from build123d import *

# Parameters (mm, degrees)
EXTRUDE_1_DEPTH = 1
SKETCH_2_R      = 3
EXTRUDE_2_DEPTH = 2
SKETCH_3_R      = 3
EXTRUDE_3_DEPTH = 2


with BuildPart() as part:
    # 草图1 → 凸台-拉伸1 (new body)
    with BuildSketch(Plane.XY):
        with BuildLine():
            Line((0, -3.874788925), (-258.053276248, -3.874788925))
            ThreePointArc((-258.053276248, -3.874788925), (-261.928065173, 0), (-258.053276248, 3.874788925))
            Line((-258.053276248, 3.874788925), (0, 3.874788925))
            ThreePointArc((0, 3.874788925), (3.874788925, 0), (0, -3.874788925))
        make_face()
    extrude(amount=EXTRUDE_1_DEPTH)

    # 草图2 → 凸台-拉伸2 (add)
    with BuildSketch(Plane.XY.offset(1)):
        Circle(SKETCH_2_R)
    extrude(amount=EXTRUDE_2_DEPTH)

    # 草图3 → 凸台-拉伸3 (add)
    with BuildSketch(Plane.XY.offset(1)):
        with Locations((-258.053276248, 0)):
            Circle(SKETCH_3_R)
    extrude(amount=EXTRUDE_3_DEPTH)


solid = part.part
Geometry: final body of the model. Coordinates: model frame, mm. A direction names the side the tool comes from. Give positions to 0.01 mm unless a question says otherwise; leave off trailing zeros. Order: outer loops, then holes, each group sorted by start corner. A loop starts at its lowest first (then second) coordinate and runs counter-clockwise, first axis right, second up. Notation, with made-up numbers: (72, 20) -> (95, 20) arc R17 ccw to (95, 24) -> close; hole circle Ø4 at (-37, 71.5). An arc over 180 degrees is marked (long way). Answer as a JSON object with one key per item and string values.
Q1. Material intervals for probe 1 along X at (y, z) = (-0.25, 2.6); probe 2 along Z at (x, y) = (-14, -0.75); probe 3 along X at (y, z) = (-0.25, 0.7), sorted ascending.
Entries:
{"probe 1": "x = -261.04 to -255.06, -2.99 to 2.99", "probe 2": "z = 0 to 1", "probe 3": "x = -261.92 to 3.87"}
Q2. Section C-C (x = -232.5). Output: boundary loops of the cut face in (y, z).
Entries:
{"outline": "(-3.87, 0) -> (3.87, 0) -> (3.87, 1) -> (-3.87, 1) -> close"}
Q3. Draft query along X for faces 3 (the flat face through (-127, 0, 0)), 4 (the cylindrical face through (-3, 0, 2)). Return one class per face: released by +X, released by -X, zero draft, split by the parting line, or undercut.
Entries:
{"face 3": "zero draft", "face 4": "undercut"}
Q4. Access query for faces 1 (the flat face through (0, 0, 3)), 2 (the cylindrical face through (-261.05, 0.13, 1.99)). Directions: +Z, -Z, +X, -X, +Y, -Y. A direction counts if a zero-diameter tool reaches every point of the face in a straight line with its end or side. Return the directions, or none.
Entries:
{"face 1": "+Z, +X, -X, +Y, -Y", "face 2": "+Z"}
Q5. Section B-B (z = 1.55). Output: boundary loops of the cut face in (x, y), plus the area to 3 significant figures.
Entries:
{"outline": "circle Ø6 at (-258.05, 0); circle Ø6 at (0, 0)", "area": "56.5 mm^2"}
Q6. Section A-A (y = 0). Output: boundary loops of the cut face in (x, z), plus the area to 3 significant figures.
Entries:
{"outline": "(-261.93, 0) -> (3.87, 0) -> (3.87, 1) -> (3, 1) -> (3, 3) -> (-3, 3) -> (-3, 1) -> (-255.05, 1) -> (-255.05, 3) -> (-261.05, 3) -> (-261.05, 1) -> (-261.93, 1) -> close", "area": "290 mm^2"}
Q7. First-contact query: pin 1 (1.5 mm diameter, centred on y = 2.5, z = 0.5, fed in from +X); pin 2 (4 mm diameter, centred on x = -176, y = -0.5, fed in from +Z). Flat tips, straight axial feed; report the tip coordinate or a pass-through.
Entries:
{"pin 1": "stops at x = 3.46", "pin 2": "stops at z = 1"}
